For this review, take the finished solid that the model builds, in its own axes (mm). Round coordinates to 2 decimals unless told otherwise and drop trailing zeros. Put each result on its own line as item: value. Start each with the question number.
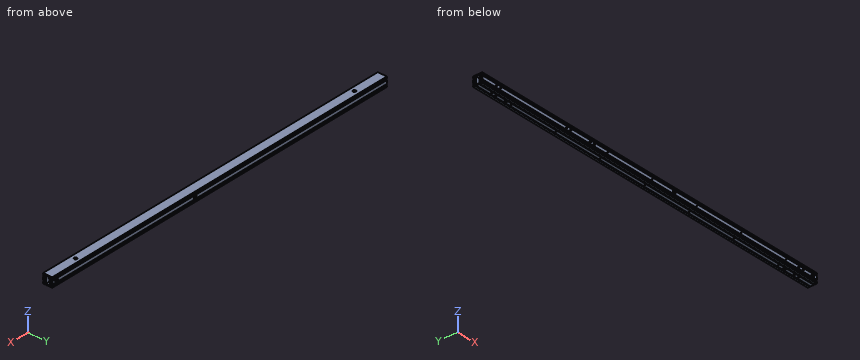
```python
from build123d import *

# Parameters (mm, degrees)
SKETCH_1_W             = 23.5
SKETCH_1_H             = 12
EXTRUDE_1_DEPTH        = 601
HOLE_WIZARD_M6_1_D     = 5
HOLE_WIZARD_M6_1_DEPTH = 15
HOLE_WIZARD_M6_1_TIP   = 1.502151548
HOLE_WIZARD_M6_2_D     = 5
HOLE_WIZARD_M6_2_DEPTH = 15
HOLE_WIZARD_M6_2_TIP   = 1.502151548
SKETCH_6_R             = 5.05
CUT_EXTRUDE_1_DEPTH    = 602.935212461
HOLE_WIZARD_M4_1_D     = 3.3
HOLE_WIZARD_M4_1_DEPTH = 10.1
HOLE_WIZARD_M4_1_TIP   = 0.991420021
SKETCH_10_R            = 4.5
CUT_EXTRUDE_2_DEPTH    = 602.935212461
HOLE_WIZARD_M4_2_D     = 3.3
HOLE_WIZARD_M4_2_DEPTH = 10.1
HOLE_WIZARD_M4_2_TIP   = 0.991420021


with BuildPart() as part:
    # 草图1 → 凸台-拉伸1 (new, symmetric)
    with BuildSketch(Plane(origin=(0, 0, 0), x_dir=(0, 0, -1), z_dir=(1, 0, 0))):
        with BuildLine():
            Line((-14, 15), (-11.5, 15))
            Line((-11.5, 15), (-11.5, 13.5))
            Line((-11.5, 13.5), (-11.4, 13.5))
            ThreePointArc((-11.4, 13.5), (-11.117157288, 13.382842712), (-11, 13.1))
            Line((-11, 13.1), (-11, 12))
            Line((-11, 12), (-9.5, 12))
            Line((-9.5, 12), (-9.5, 15))
            Line((-9.5, 15), (-8, 15))
            Line((-8, 15), (-8, 12.5))
            Line((-8, 12.5), (-5, 12.5))
            Line((-5, 12.5), (-5, 15))
            Line((-5, 15), (5, 15))
            Line((5, 15), (5, 12.5))
            Line((5, 12.5), (8, 12.5))
            Line((8, 12.5), (8, 15))
            Line((8, 15), (9.5, 15))
            Line((9.5, 15), (9.5, 12))
            Line((9.5, 12), (11, 12))
            Line((11, 12), (11, 13.1))
            ThreePointArc((11, 13.1), (11.117157288, 13.382842712), (11.4, 13.5))
            Line((11.4, 13.5), (11.5, 13.5))
            Line((11.5, 13.5), (11.5, 15))
            Line((11.5, 15), (14, 15))
            ThreePointArc((14, 15), (14.707106781, 14.707106781), (15, 14))
            Line((15, 14), (15, 8))
            Line((15, 8), (12.5, 8))
            Line((12.5, 8), (12.5, 5))
            Line((12.5, 5), (15, 5))
            Line((15, 5), (15, -5))
            Line((15, -5), (12.5, -5))
            Line((12.5, -5), (12.5, -8))
            Line((12.5, -8), (15, -8))
            Line((15, -8), (15, -14))
            ThreePointArc((15, -14), (14.707106781, -14.707106781), (14, -15))
            Line((14, -15), (11.5, -15))
            Line((11.5, -15), (11.5, -13.5))
            Line((11.5, -13.5), (11.4, -13.5))
            ThreePointArc((11.4, -13.5), (11.117157288, -13.382842712), (11, -13.1))
            Line((11, -13.1), (11, -12))
            Line((11, -12), (9.5, -12))
            Line((9.5, -12), (9.5, -15))
            Line((9.5, -15), (8, -15))
            Line((8, -15), (8, -12.5))
            Line((8, -12.5), (5, -12.5))
            Line((5, -12.5), (5, -15))
            Line((5, -15), (-5, -15))
            Line((-5, -15), (-5, -12.5))
            Line((-5, -12.5), (-8, -12.5))
            Line((-8, -12.5), (-8, -15))
            Line((-8, -15), (-9.5, -15))
            Line((-9.5, -15), (-9.5, -12))
            Line((-9.5, -12), (-11, -12))
            Line((-11, -12), (-11, -13.1))
            ThreePointArc((-11, -13.1), (-11.117157288, -13.382842712), (-11.4, -13.5))
            Line((-11.4, -13.5), (-11.5, -13.5))
            Line((-11.5, -13.5), (-11.5, -15))
            Line((-11.5, -15), (-14, -15))
            ThreePointArc((-14, -15), (-14.707106781, -14.707106781), (-15, -14))
            Line((-15, -14), (-15, 14))
            ThreePointArc((-15, 14), (-14.707106781, 14.707106781), (-14, 15))
        make_face()
        with BuildLine():
            Line((12, -10.5), (12, -8.5))
            ThreePointArc((12, -8.5), (11.853553391, -8.146446609), (11.5, -8))
            Line((11.5, -8), (-11.5, -8))
            ThreePointArc((-11.5, -8), (-11.853553391, -8.146446609), (-12, -8.5))
            Line((-12, -8.5), (-12, -10.5))
            ThreePointArc((-12, -10.5), (-11.853553391, -10.853553391), (-11.5, -11))
            Line((-11.5, -11), (11.5, -11))
            ThreePointArc((11.5, -11), (11.853553391, -10.853553391), (12, -10.5))
        make_face(mode=Mode.SUBTRACT)
        with BuildLine():
            Line((-11.5, 11), (11.5, 11))
            ThreePointArc((11.5, 11), (11.853553391, 10.853553391), (12, 10.5))
            Line((12, 10.5), (12, 8.5))
            ThreePointArc((12, 8.5), (11.853553391, 8.146446609), (11.5, 8))
            Line((11.5, 8), (-11.5, 8))
            ThreePointArc((-11.5, 8), (-11.853553391, 8.146446609), (-12, 8.5))
            Line((-12, 8.5), (-12, 10.5))
            ThreePointArc((-12, 10.5), (-11.853553391, 10.853553391), (-11.5, 11))
        make_face(mode=Mode.SUBTRACT)
        Rectangle(SKETCH_1_W, SKETCH_1_H, mode=Mode.SUBTRACT)
    extrude(amount=EXTRUDE_1_DEPTH, both=True)

    # M6 螺纹孔1
    with Locations(Plane(origin=(0, 0, -15), x_dir=(-1, 0, 0), z_dir=(0, 0, -1))):
        with Locations((-551, 0), (-536, 0), (536, 0), (551, 0)):
            Hole(HOLE_WIZARD_M6_1_D / 2, depth=HOLE_WIZARD_M6_1_DEPTH)
            with Locations((0, 0, -(HOLE_WIZARD_M6_1_DEPTH + HOLE_WIZARD_M6_1_TIP / 2))):  # 118° drill point
                Cone(0, HOLE_WIZARD_M6_1_D / 2, HOLE_WIZARD_M6_1_TIP, mode=Mode.SUBTRACT)

    # M6 螺纹孔2
    with Locations(Plane.XZ.offset(15)):
        with Locations((551, 0), (536, 0), (-199, 0), (-214, 0), (-284, 0), (-299, 0), (-536, 0), (-551, 0)):
            Hole(HOLE_WIZARD_M6_2_D / 2, depth=HOLE_WIZARD_M6_2_DEPTH)
            with Locations((0, 0, -(HOLE_WIZARD_M6_2_DEPTH + HOLE_WIZARD_M6_2_TIP / 2))):  # 118° drill point
                Cone(0, HOLE_WIZARD_M6_2_D / 2, HOLE_WIZARD_M6_2_TIP, mode=Mode.SUBTRACT)

    # 草图6 → 切除-拉伸1 (cut, through all)
    with BuildSketch(Plane.XZ.offset(15)):
        with Locations(Location((88, 0, 0), (0, 0, 90))):
            Circle(SKETCH_6_R)
        with Locations(Location((586, 0, 0), (0, 0, 90))):
            Circle(SKETCH_6_R)
    extrude(amount=-CUT_EXTRUDE_1_DEPTH, mode=Mode.SUBTRACT)

    # M4 螺纹孔1
    with Locations(Plane.XZ.offset(15)):
        with Locations((489, 0), (329, 0), (169, 0), (9, 0), (-151, 0)):
            Hole(HOLE_WIZARD_M4_1_D / 2, depth=HOLE_WIZARD_M4_1_DEPTH)
            with Locations((0, 0, -(HOLE_WIZARD_M4_1_DEPTH + HOLE_WIZARD_M4_1_TIP / 2))):  # 118° drill point
                Cone(0, HOLE_WIZARD_M4_1_D / 2, HOLE_WIZARD_M4_1_TIP, mode=Mode.SUBTRACT)

    # 草图10 → 切除-拉伸2 (cut, through all)
    with BuildSketch(Plane.XY.offset(15)):
        with Locations((-501, 0)):
            Circle(SKETCH_10_R)
        with Locations((501, 0)):
            Circle(SKETCH_10_R)
    extrude(amount=-CUT_EXTRUDE_2_DEPTH, mode=Mode.SUBTRACT)

    # M4 螺纹孔2
    with Locations(Plane(origin=(0, 0, -15), x_dir=(-1, 0, 0), z_dir=(0, 0, -1))):
        with Locations((-479, 0), (-319, 0), (-159, 0), (1, 0), (161, 0), (321, 0), (481, 0)):
            Hole(HOLE_WIZARD_M4_2_D / 2, depth=HOLE_WIZARD_M4_2_DEPTH)
            with Locations((0, 0, -(HOLE_WIZARD_M4_2_DEPTH + HOLE_WIZARD_M4_2_TIP / 2))):  # 118° drill point
                Cone(0, HOLE_WIZARD_M4_2_D / 2, HOLE_WIZARD_M4_2_TIP, mode=Mode.SUBTRACT)


solid = part.part
```
Item 1: Insertion check: pin 1 Ø2 at (x, z) = (-471, -6.5) entering from -Y; pin 2 Ø3 at (x, y) = (479, 0) entering from -Z. Each pin has a flat end and moves straight along its axis. Give the tip position at first contact, or say it passes through.
Item 2: Consider section A-A, the plane x = 204. Count the separate pieces of the cut face and the enclosed holes in it, plus the area to 3 significant figures.
Item 3: For L1, parallel to Y at x = 238, z = -6; L2, parallel to Y at x = -470.5, z = 0; L3, parallel to Z at x = 169, y = -13, list the stretches that pass through material, from the lowest coordinate up.
Evaluation:
1. pin 1: stops at y = -12.5
1. pin 2: stops at z = 11.75
2. separate pieces: 1
2. enclosed holes: 3
2. area: 407 mm^2
3. L1: y = -12.5 to -11, -8 to -6, 6 to 8, 11 to 12.5
3. L2: y = -15 to -11, -8 to -6, 6 to 8, 11 to 15
3. L3: z = -15 to -11, -9.5 to -8, -5 to -1.65, 1.65 to 5, 8 to 9.5, 11 to 15
